For this review, take the finished solid that the model builds, in its own axes (mm). Face numbers are marked on the shaded views. A direction names the side the tool comes from. Give positions to 0.01 mm unless a question says otherwise; leave off trailing zeros. Order: outer loops, then holes, each group sorted by start corner. A loop starts at its lowest first (then second) coordinate and runs counter-clockwise, first axis right, second up. Notation, with made-up numbers: (16.5, 63.5) -> (21.5, 63.5) arc R25 cw to (21.5, 89.5) -> close; hole circle Ø5 at (68, 5). An arc over 180 degrees is marked (long way). Return JSON: item names as keys, results as strings. Group by question number.
1) Add section D-D (x = -6). Give the boundary of the cut face in (y, z).
2) Add section C-C (z = 6.25). Give the boundary of the cut face in (x, y), then the cut area to 3 significant figures.
3) Insertion check: P1, Ø1, axis at y = 22, z = -3.5, coming from the -X side; P2, Ø1.5, axis at x = 3.5, y = 15, coming from the -Z side; P3, Ø4, axis at x = 5.5, y = 23.5, coming from the -Z side. Each pin has a flat end and moves straight along its axis. Give the tip position at first contact, or say it passes through.
4) To check wall thickness, follow line 1 along Z through (x, y) = (0, 6) (1 decimal); line 2 along X through (y, z) = (48, 0). State the ranges of each line that lie inside material, in increasing order.
5) Add section B-B (y = 34). Give the boundary of the cut face in (x, z) (1 decimal), then the cut area to 3 significant figures.
6) The part is to be moulded in two halves that separate along Z. For the marked faces 1, 2 and 3, say which applies: released by +Z, released by -Z, zero draft, split by the parting line, or undercut.
7) For the marked faces 4 and 5, list the 3-axis set-ups (+Z, -Z, +X, -X, +Y, -Y) from which the entire face can be reached by the end or side of a thin tool; tool diameter is ignored.
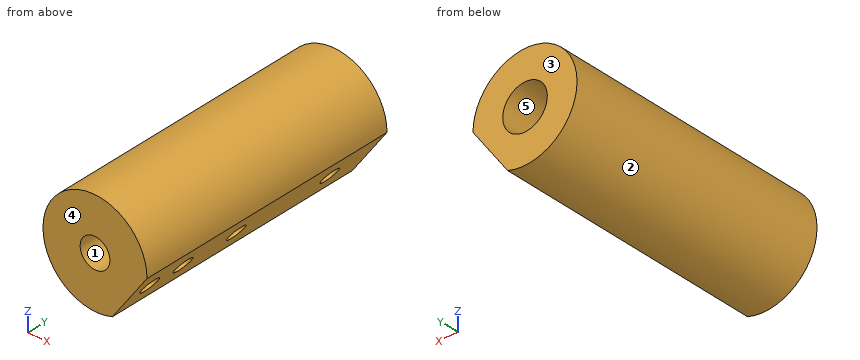
from build123d import *

# Parameters (mm, degrees)
SKETCH1_R               = 11.1125
SKETCH1_R_2             = 3.175
BOSS_EXTRUDE1_DEPTH     = 57.15
CUT_EXTRUDE2_DEPTH      = 60.271391181
CUT_EXTRUDE2_DEPTH_BACK = 57.15
SKETCH3_R               = 4.7625
CUT_EXTRUDE3_DEPTH      = 38.1
CUT_EXTRUDE4_REACH      = 64.262
SKETCH4_R               = 1.984375


with BuildPart() as part:
    # Sketch1 → Boss-Extrude1 (new body)
    with BuildSketch(Plane(origin=(0, 0, 0), x_dir=(1, 0, 0), z_dir=(0, 1, 0))):
        with Locations(Location((0, 0, 0), (0, 0, 270))):
            Circle(SKETCH1_R)
        with Locations(Location((0, 0, 0), (0, 0, 270))):
            Circle(SKETCH1_R_2, mode=Mode.SUBTRACT)
    extrude(amount=BOSS_EXTRUDE1_DEPTH)

    # Sketch2 → Cut-Extrude2 (cut, two sides: drawn at the far end of the back side and taken through both)
    with BuildSketch(Plane(origin=(0, 57.15, 0), x_dir=(1, 0, 0), z_dir=(0, 1, 0)).offset(-CUT_EXTRUDE2_DEPTH_BACK)):
        Polygon((-32.277943168, 61.417010445), (3.712797685, 10.473909948), (11.1125, 0), (47.103240854, -50.943100497), (148.989441847, 21.03838121), (69.608257825, 133.398492152), align=None)
    extrude(amount=CUT_EXTRUDE2_DEPTH + CUT_EXTRUDE2_DEPTH_BACK, mode=Mode.SUBTRACT)

    # Sketch3 → Cut-Extrude3 (cut)
    with BuildSketch(Plane(origin=(0, 57.15, 0), x_dir=(1, 0, 0), z_dir=(0, 1, 0))):
        with Locations(Location((0, 0, 0), (0, 0, 270))):
            Circle(SKETCH3_R)
    extrude(amount=-CUT_EXTRUDE3_DEPTH, mode=Mode.SUBTRACT)

    # Sketch4 → Cut-Extrude4 (cut, up to next)
    with BuildSketch(Plane(origin=(7.412648843, 0, -5.236954974), x_dir=(-0.5770138525497868, 0, -0.8167343594863956), z_dir=(0.8167343594863956, 0, -0.5770138525497868)), mode=Mode.PRIVATE) as cut_extrude4_sk1:
        with Locations((0, 47.625)):
            Circle(SKETCH4_R)
    cut_extrude4_tool1 = extrude(cut_extrude4_sk1.sketch, amount=-CUT_EXTRUDE4_REACH, mode=Mode.PRIVATE) & part.part
    # Sketch4 → Cut-Extrude4 (cut, up to next)
    with BuildSketch(Plane(origin=(7.412648843, 0, -5.236954974), x_dir=(-0.5770138525497868, 0, -0.8167343594863956), z_dir=(0.8167343594863956, 0, -0.5770138525497868)), mode=Mode.PRIVATE) as cut_extrude4_sk2:
        with Locations((0, 25.4)):
            Circle(SKETCH4_R)
    cut_extrude4_tool2 = extrude(cut_extrude4_sk2.sketch, amount=-CUT_EXTRUDE4_REACH, mode=Mode.PRIVATE) & part.part
    # Sketch4 → Cut-Extrude4 (cut, up to next)
    with BuildSketch(Plane(origin=(7.412648843, 0, -5.236954974), x_dir=(-0.5770138525497868, 0, -0.8167343594863956), z_dir=(0.8167343594863956, 0, -0.5770138525497868)), mode=Mode.PRIVATE) as cut_extrude4_sk3:
        with Locations((0, 12.7)):
            Circle(SKETCH4_R)
    cut_extrude4_tool3 = extrude(cut_extrude4_sk3.sketch, amount=-CUT_EXTRUDE4_REACH, mode=Mode.PRIVATE) & part.part
    # Sketch4 → Cut-Extrude4 (cut, up to next)
    with BuildSketch(Plane(origin=(7.412648843, 0, -5.236954974), x_dir=(-0.5770138525497868, 0, -0.8167343594863956), z_dir=(0.8167343594863956, 0, -0.5770138525497868)), mode=Mode.PRIVATE) as cut_extrude4_sk4:
        with Locations((0, 4.7625)):
            Circle(SKETCH4_R)
    cut_extrude4_tool4 = extrude(cut_extrude4_sk4.sketch, amount=-CUT_EXTRUDE4_REACH, mode=Mode.PRIVATE) & part.part
    add(cut_extrude4_tool1.solids().sort_by_distance((7.412649, 47.625, -5.236955))[0], mode=Mode.SUBTRACT)
    add(cut_extrude4_tool2.solids().sort_by_distance((7.412649, 25.4, -5.236955))[0], mode=Mode.SUBTRACT)
    add(cut_extrude4_tool3.solids().sort_by_distance((7.412649, 12.7, -5.236955))[0], mode=Mode.SUBTRACT)
    add(cut_extrude4_tool4.solids().sort_by_distance((7.412649, 4.7625, -5.236955))[0], mode=Mode.SUBTRACT)


solid = part.part
Evaluation:
{
 "1": {"outline": "(0, -9.35) -> (57.15, -9.35) -> (57.15, 9.35) -> (0, 9.35) -> close"},
 "2": {"outline": "(-9.19, 0) -> (9.19, 0) -> (9.19, 57.15) -> (-9.19, 57.15) -> close", "area": "1,050 mm^2"},
 "3": {"P1": "x = -10.7", "P2": "z = -10.77", "P3": "z = -10.55"},
 "4": {"line 1": "-11.1 to -3.2, 3.2 to 11.1", "line 2": "-11.11 to -4.76, 4.76 to 11.11"},
 "5": {"outline": "(3.7, -10.5) -> (11.1, 0) arc R11.1 ccw (long way) to start; hole circle Ø9.5 at (0, 0)", "area": "299 mm^2"},
 "6": {"face 1": "undercut", "face 2": "split by the parting line", "face 3": "zero draft"},
 "7": {"face 4": "+Z, -Z, +X, -X, -Y", "face 5": "+Y"}
}
